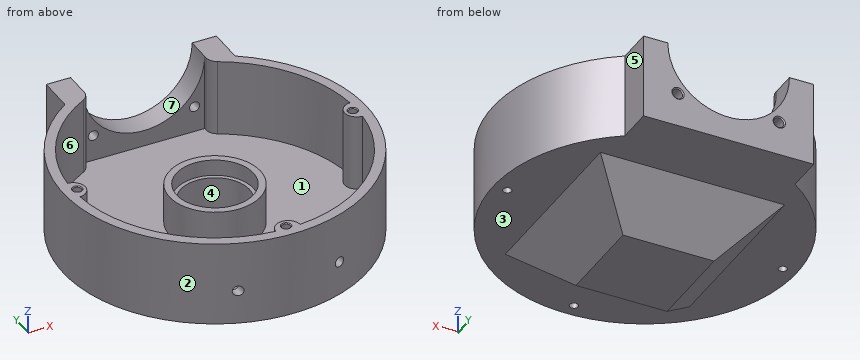
```python
from build123d import *

# Parameters (mm, degrees)
EXTRUDE_1_DEPTH              = 42
CUT_EXTRUDE_1_DEPTH          = 38
HOLE_WIZARD_M5_1_D           = 4.2
HOLE_WIZARD_M5_1_CSINK_D     = 5.05
HOLE_WIZARD_M5_1_CSINK_ANGLE = 90
PATTERN_CIRCULAR_1_COUNT     = 4
CUT_EXTRUDE_3_REACH          = 119.427
SKETCH_6_R                   = 30
HOLE_WIZARD_M6_1_D           = 5
HOLE_WIZARD_M6_1_CSINK_D     = 6.05
HOLE_WIZARD_M6_1_CSINK_ANGLE = 90
SKETCH_9_W                   = 91
SKETCH_9_H                   = 91
EXTRUDE_2_DEPTH              = 23
EXTRUDE_2_TAPER              = 45
SKETCH_10_R                  = 22.5
EXTRUDE_3_DEPTH              = 20
SKETCH_11_R                  = 19
CUT_EXTRUDE_4_DEPTH          = 8
SKETCH_12_R                  = 17
CUT_EXTRUDE_5_DEPTH          = 32


with BuildPart() as part:
    # 草图1 → 凸台-拉伸1 (new body)
    with BuildSketch(Plane.XY):
        with BuildLine():
            Line((-42, 62.136945532), (-42, 80))
            Line((-42, 80), (42, 80))
            Line((42, 80), (42, 62.136945532))
            ThreePointArc((42, 62.136945532), (0, -75), (-42, 62.136945532))
        make_face()
    extrude(amount=EXTRUDE_1_DEPTH)

    # 草图2 → 切除-拉伸1 (cut)
    with BuildSketch(Plane.XY.offset(42)):
        with BuildLine():
            Line((-30, 66.932802123), (-30, 68))
            Line((-30, 68), (30, 68))
            Line((30, 68), (30, 66.932802123))
            ThreePointArc((30, 66.932802123), (30.849629548, 63.854867066), (33.157894737, 61.648633534))
            ThreePointArc((33.157894737, 61.648633534), (58.493479839, 38.451434516), (69.742857143, 5.994487263))
            ThreePointArc((69.742857143, 5.994487263), (64, 0), (69.742857143, -5.994487263))
            ThreePointArc((69.742857143, -5.994487263), (49.497474683, -49.497474683), (5.994487263, -69.742857143))
            ThreePointArc((5.994487263, -69.742857143), (0, -64), (-5.994487263, -69.742857143))
            ThreePointArc((-5.994487263, -69.742857143), (-49.497474683, -49.497474683), (-69.742857143, -5.994487263))
            ThreePointArc((-69.742857143, -5.994487263), (-64, 0), (-69.742857143, 5.994487263))
            ThreePointArc((-69.742857143, 5.994487263), (-58.493479839, 38.451434516), (-33.157894737, 61.648633534))
            ThreePointArc((-33.157894737, 61.648633534), (-30.849629548, 63.854867066), (-30, 66.932802123))
        make_face()
    extrude(amount=-CUT_EXTRUDE_1_DEPTH, mode=Mode.SUBTRACT)

    # M5 螺纹孔1 (through all)
    with Locations(Plane.XY.offset(42)):
        with Locations((0, -68)):
            hole_wizard_m5_1 = CounterSinkHole(HOLE_WIZARD_M5_1_D / 2, HOLE_WIZARD_M5_1_CSINK_D / 2, counter_sink_angle=HOLE_WIZARD_M5_1_CSINK_ANGLE)

    # 阵列(圆周)1: M5 螺纹孔1 ×4 about axis, 1 skipped
    pattern_circular_1_axis = Axis((0, 0, 0), (0, 0, -1))
    add([hole_wizard_m5_1.rotate(pattern_circular_1_axis, i * 360 / PATTERN_CIRCULAR_1_COUNT) for i in range(1, PATTERN_CIRCULAR_1_COUNT) if i not in (2,)], mode=Mode.SUBTRACT)

    # 草图6 → 切除-拉伸3 (cut, up to next)
    with BuildSketch(Plane(origin=(0, 0, 0), x_dir=(1, 0, 0), z_dir=(0, 1, 0)), mode=Mode.PRIVATE) as cut_extrude_3_sk1:
        with Locations((0, -42)):
            Circle(SKETCH_6_R)
    cut_extrude_3_tool1 = extrude(cut_extrude_3_sk1.sketch, amount=CUT_EXTRUDE_3_REACH, mode=Mode.PRIVATE) & part.part
    add(cut_extrude_3_tool1.solids().sort_by_distance((0, 0, 42))[0], mode=Mode.SUBTRACT)

    # M6 螺纹孔1 (through all)
    with Locations(Plane(origin=(0, 80, 0), x_dir=(1, 0, 0), z_dir=(0, 1, 0))):
        with Locations((25, -17), (-25, -17)):
            CounterSinkHole(HOLE_WIZARD_M6_1_D / 2, HOLE_WIZARD_M6_1_CSINK_D / 2, counter_sink_angle=HOLE_WIZARD_M6_1_CSINK_ANGLE)

    # 草图9 → 凸台-拉伸2 (add)
    with BuildSketch(Plane(origin=(0, 0, 0), x_dir=(-1, 0, 0), z_dir=(0, 0, -1))):
        Rectangle(SKETCH_9_W, SKETCH_9_H)
    extrude(amount=EXTRUDE_2_DEPTH, taper=EXTRUDE_2_TAPER)

    # 草图10 → 凸台-拉伸3 (add)
    with BuildSketch(Plane.XY.offset(4)):
        Circle(SKETCH_10_R)
    extrude(amount=EXTRUDE_3_DEPTH)

    # 草图11 → 切除-拉伸4 (cut)
    with BuildSketch(Plane.XY.offset(24)):
        Circle(SKETCH_11_R)
    extrude(amount=-CUT_EXTRUDE_4_DEPTH, mode=Mode.SUBTRACT)

    # 草图12 → 切除-拉伸5 (cut)
    with BuildSketch(Plane.XY.offset(16)):
        Circle(SKETCH_12_R)
    extrude(amount=-CUT_EXTRUDE_5_DEPTH, mode=Mode.SUBTRACT)


solid = part.part
```
Input: part model. Units: mm. Frame: model coordinates. Face numbers are marked on the shaded views. A direction names the side the tool comes from. Round coordinates to 2 decimals unless told otherwise and drop trailing zeros. Loops run counter-clockwise (first coordinate to the right, second up) from the corner with the lowest first, then second, coordinate; pieces in that order, holes last. Notation, with made-up numbers: (61, 6) -> (92, 6) arc R16 cw to (92, 34) -> close; hole circle Ø9 at (76.25, 12.25). An arc over 180 degrees is marked (long way). One line per item, written item: value.
(1) Mould query, pull axis X, two halves, no side actions, for the marked faces 1, 2, 3 and 4. Classes: pulls with the +X half, pulls with the -X half, needs draft (parallel to the pull), parting line crosses it, or undercut.
Geometry check:
face 1: undercut
face 2: parting line crosses it
face 3: needs draft
face 4: undercut
(2) Set-up query: the marked faces 5, 6 and 7. Return all of +Z, -Z, +X, -X, +Y, -Y with unobstructed straight access to the full face (end or side cutting, diameter ignored); none if empty.
Geometry check:
face 5: +Z, -Z, +X, +Y
face 6: +Z
face 7: +Z, +Y
(3) Material intervals for line 1 (X direction, y = 71, z = 17); line 2 (X direction, y = -19.5, z = 9); line 3 (Y direction, x = 60, z = 8), sorted ascending. Write a range as [from, to].
Geometry check:
line 1: [-42, -27.5], [-22.5, -16.58], [16.58, 22.5], [27.5, 42]
line 2: [-72.42, -67.23], [-11.22, 11.22], [67.23, 72.42]
line 3: [-45, -36.06], [36.06, 45]
(4) Pin query (flat end, axial travel): pin 1 (3 mm diameter, centred on x = 26, y = -19, fed in from +Z); pin 2 (3 mm diameter, centred on x = 1, y = -49.5, fed in from -Z); pin 3 (9 mm diameter, centred on y = 72.5, z = 21, fed in from +X); pin 4 (4.5 mm diameter, centred on x = 25, z = 17, fed in from +Y). Return the tip coordinate at first contact, or that it passes through.
Geometry check:
pin 1: z = 4
pin 2: z = 0
pin 3: x = 42
pin 4: through
(5) Section C-C (y = -59.5). Return the cut outline in (x, z).
Geometry check:
outline: (-45.66, 0) -> (45.66, 0) -> (45.66, 42) -> (36.87, 42) -> (36.87, 4) -> (-36.87, 4) -> (-36.87, 42) -> (-45.66, 42) -> close
(6) Section B-B (z = 30). Return the cut outline in (x, y), plus the area to 3 significant figures.
Geometry check:
outline: (-69.74, -5.99) arc R6 ccw to (-69.74, 5.99) arc R70 cw to (-33.16, 61.65) arc R6 ccw to (-30, 66.93) -> (-30, 68) -> (-27.5, 68) -> (-27.5, 80) -> (-42, 80) -> (-42, 62.14) arc R75 ccw (long way) to (42, 62.14) -> (42, 80) -> (27.5, 80) -> (27.5, 68) -> (30, 68) -> (30, 66.93) arc R6 ccw to (33.16, 61.65) arc R70 cw to (69.74, 5.99) arc R6 ccw to (69.74, -5.99) arc R70 cw to (5.99, -69.74) arc R6 ccw to (-5.99, -69.74) arc R70 cw to start; hole circle Ø4.2 at (-68, 0); hole circle Ø4.2 at (0, -68); hole circle Ø4.2 at (68, 0)
area: 2,490 mm2
(7) Section A-A (y = 0). Give the number of separate pieces and of enclosed holes in the cut face, plus the area to 3 significant figures.
Geometry check:
separate pieces: 3
enclosed holes: 0
area: 2,150 mm2
